from build123d import *

# Parameters (mm, degrees)
F1_DEPTH = 406.4
F2_R     = 25.88143
F3_DEPTH = 762
F4_R     = 25.4
F5_DEPTH = 1524
F6_R     = 25.67789
F7_DEPTH = 45.72


with BuildPart() as f1:
    # F0 (on Front) → F1 (new body)
    with BuildSketch(Plane.XZ):
        Polygon((43.292664, -76.169349), (87.610923, -0.592128), (44.318259, 75.577221), (-43.292664, 76.169349), (-87.610923, 0.592128), (-44.318259, -75.577221), align=None)
    extrude(amount=F1_DEPTH)

    # F2 (on Right) → F3 (join)
    with BuildSketch(Plane.YZ):
        with Locations((-182.547286, 0)):
            Circle(F2_R)
    extrude(amount=F3_DEPTH)

    # F4 (on Right) → F5 (join)
    with BuildSketch(Plane.YZ):
        with Locations((-174.269957, 0)):
            Circle(F4_R)
    extrude(amount=-F5_DEPTH)

    # F6 (on Front) → F7 (join)
    with BuildSketch(Plane.XZ):
        Circle(F6_R)
    extrude(amount=-F7_DEPTH)


solid = f1.part
Geometry check sheet. Reference: the model listing, model coordinates, mm. A direction names the side the tool comes from. Give positions to 0.01 mm unless a question says otherwise; leave off trailing zeros. Loops run counter-clockwise (first coordinate to the right, second up) from the corner with the lowest first, then second, coordinate; pieces in that order, holes last.
(1) Section check B-B on x = 0. Record the cut outline in (y, z), then the cut area to 3 significant figures.
From the geometry:
outline: (-406.4, -75.88) - (0, -75.88) - (0, -25.68) - (45.72, -25.68) - (45.72, 25.68) - (0, 25.68) - (0, 75.88) - (-406.4, 75.88) - close
area: 64,000 mm2
(2) Thickness scan on L1, parallel to Y at x = -779, z = 0; L2, parallel to X at y = -291, z = 26; L3, parallel to Y at x = 519, z = 21. Record the ranges inside material, lowest first.
From the geometry:
L1: y = -199.67 to -148.87
L2: x = -72.71 to 72.5
L3: y = -197.68 to -167.42
(3) Depth check by flat-ended pin: pin 1 Ø2 at (x, z) = (-306, -0.5) entering from -Y; pin 2 Ø6 at (x, y) = (-22, -44.5) entering from +Z; pin 3 Ø10 at (y, z) = (-246, 57.5) entering from -X. Enter the tip coordinate at first touch or a pass-through.
From the geometry:
pin 1: stops at y = -199.67
pin 2: stops at z = 76.05
pin 3: stops at x = -57.17
(4) Set-up check for faces 1 (the flat face through (66.268, -200.355, 36.959)), 2 (the flat face through (-66.268, -200.355, -36.959)), 3 (the flat face through (65.14, -200.36, -38.91)), 4 (the flat face through (-65.14, -200.36, 38.91)), 5 (the cylindrical face through (-3.34, 22.54, 25.46)): record each of +Z, -Z, +X, -X, +Y, -Y from which the full face is reachable in a straight line by a thin tool's end or side.
From the geometry:
face 1: +Z, +X
face 2: -Z, -X
face 3: -Z, +X
face 4: +Z, -X
face 5: +Y
(5) Section check A-A on y = -350.5. Record the cut outline in (x, z), then the cut area to 3 significant figures.
From the geometry:
outline: (-87.61, 0.59) - (-44.32, -75.58) - (43.29, -76.17) - (87.61, -0.59) - (44.32, 75.58) - (-43.29, 76.17) - close
area: 19,900 mm2
(6) Section check D-D on x = -1073. Record the cut outline in (y, z), then the cut area to 3 significant figures.
From the geometry:
outline: circle Ø50.8 at (-174.27, 0)
area: 2,030 mm2
(7) Section check C-C on x = 518. Record the cut outline in (y, z), then the cut area to 3 significant figures.
From the geometry:
outline: circle Ø51.76 at (-182.55, 0)
area: 2,100 mm2
